```python
from build123d import *

# Parameters (mm, degrees)
PAD047_DEPTH      = 4
SKETCH067_R       = 4.5
PAD048_DEPTH      = 22
PAD049_DEPTH      = 4
PAD049_DEPTH_BACK = 17


with BuildPart() as part:
    # Sketch066 → Pad047 (new body)
    with BuildSketch(Plane.YZ):
        with BuildLine():
            Line((-33, 33.999821), (-33, 45))
            Line((-33, 45), (33, 45))
            Line((33, 45), (33, 33.999804))
            ThreePointArc((24, 34), (28.499902, 29.5), (33, 33.999804))
            Line((24, 34), (24, 43))
            Line((24, 43), (-24, 43))
            Line((-24, 43), (-24, 34))
            ThreePointArc((-33, 33.999821), (-28.499911, 29.5), (-24, 34))
        make_face()
    extrude(amount=PAD047_DEPTH)

    # Sketch067 → Pad048 (join)
    with BuildSketch(Plane.YZ):
        with Locations((-28.5, 34)):
            Circle(SKETCH067_R)
        with Locations((28.5, 34)):
            Circle(SKETCH067_R)
    extrude(amount=-PAD048_DEPTH)

    # Sketch068 → Pad049 (join, two sides)
    with BuildSketch(Plane.YZ) as pad049_sk:
        Polygon((-33, 45), (-33, 43), (33, 43), (33, 45), (28.5, 49.5), (24, 45), (-24, 45), (-28.5, 49.5), align=None)
    extrude(amount=PAD049_DEPTH)
    extrude(pad049_sk.sketch, amount=-PAD049_DEPTH_BACK)


with BuildPart() as part_1:
    # Body031 placement: moved
    add(part.part.moved(Location((46, 0, 0))))


solid = part_1.part
```
The listing builds one solid part. Answer for the finished solid, in the listing's coordinates (mm). A direction names the side the tool comes from. Coordinates: 2 decimals unless noted, no trailing zeros. Write each loop counter-clockwise with the first axis right and the second up, starting at its lowest first coordinate (ties: lowest second). Pieces come first, ordered by that corner, then holes. Notation, with made-up numbers: (4, 44) - (62, 44) arc R20 ccw to (62, 66) - close; hole circle Ø5 at (27.25, 89.5). An arc over 180 degrees is marked (long way). One line per item, written item: value.
1) For a pull along Y with two mould halves and no side action, classify faces 1 (the flat face through (40, 26, 47)), 2 (the flat face through (48, -24, 39)), 3 (the flat face through (24, 28, 34)), 4 (the flat face through (44.3, -33, 43.2)) as pulls with the +Y half, pulls with the -Y half, needs draft (parallel to the pull), parting line crosses it, or undercut.
Geometry check:
face 1: undercut
face 2: undercut
face 3: needs draft
face 4: pulls with the -Y half
2) Find section D-D (y = -13.5). Give the vertices of the cut face in (x, z).
Geometry check:
outline: (29, 43) - (50, 43) - (50, 45) - (29, 45) - close
3) Find section C-C (x = 28.25). Give the vertices of the cut face in (y, z).
Geometry check:
outline: circle Ø9 at (-28.5, 34); circle Ø9 at (28.5, 34)
4) Find section B-B (z = 37.75). Give the vertices of the cut face in (x, y).
Geometry check:
outline: (24, -30.99) - (46, -30.99) - (46, -33) - (50, -33) - (50, -24) - (46, -24) - (46, -26.01) - (24, -26.01) - close; (24, 26.01) - (46, 26.01) - (46, 24) - (50, 24) - (50, 33) - (46, 33) - (46, 30.99) - (24, 30.99) - close
5) Each of these flat-tipped pins is pushed along its axis until it touches: pin 1 Ø6 at (x, y) = (32.5, 0) entering from -Z; pin 2 Ø2 at (y, z) = (-5, 47.5) entering from -X; pin 3 Ø2 at (x, z) = (30, 46.5) entering from -Y; pin 4 Ø10.5 at (x, y) = (34.5, -9) entering from +Z. Where does it stop, or does it pass through?
Geometry check:
pin 1: stops at z = 43
pin 2: passes through
pin 3: stops at y = -32.5
pin 4: stops at z = 45
6) Consider line 1 along Z through (x, y) = (47.25, -7); line 2 along X through (y, z) = (23, 44); line 3 along Y through (x, z) = (46.25, 33.5). Determine where each line is inside the solid, lowest interval first. Write a range as from..to.
Geometry check:
line 1: z = 43..45
line 2: x = 29..50
line 3: y = -32.97..-24.03, 24.03..32.97
7) A tool of negligible diameter and unlimited length cuts with its end or side. For faces 5 (the flat face through (40, 0, 43)), 6 (the flat face through (29, 0, 44)), 7 (the flat face through (48, 24, 38)), 8 (the flat face through (40, -26, 47)), 9 (the flat face through (24, -29, 34)), from which of +Z, -Z, +X, -X, +Y, -Y can it reach the whole face along a straight path? Write none if from no direction.
Geometry check:
face 5: -X
face 6: +Z, -X, +Y, -Y
face 7: -Z, +X, -X
face 8: +Z, +X, -X
face 9: +Z, -Z, -X, +Y, -Y
8) Find section A-A (x = 34.75). Give the vertices of the cut face in (y, z), and give its area (3 significant figures).
Geometry check:
outline: circle Ø9 at (-28.5, 34); (-33, 43) - (33, 43) - (33, 45) - (28.5, 49.5) - (24, 45) - (-24, 45) - (-28.5, 49.5) - (-33, 45) - close; circle Ø9 at (28.5, 34)
area: 300 mm2
